Input: part model. Units: mm. Frame: model coordinates. A direction names the side the tool comes from. Coordinates: 2 decimals unless noted, no trailing zeros. Loops run counter-clockwise (first coordinate to the right, second up) from the corner with the lowest first, then second, coordinate; pieces in that order, holes last.
(1) Contact query for flat-ended pins moving along their axis: P1, Ø1.8, axis at x = -153, y = 100, coming from the +Z side; P2, Ø3, axis at x = -121, z = 4, coming from the -Y side; P3, Ø1.8, axis at x = -77.5, z = 4, coming from the +Y side. Output: stop coordinate, or through.
(2) Set-up query: faces 5 (the face through (-67, 273, 3)), 6 (the face through (-162, 136, 3)), 7 (the face through (-120, 6, 3)), 8 (the face through (-135, 96, 3)), 9 (the face through (-110.7, 271.7, 3)). Return all of +Z, -Z, +X, -X, +Y, -Y with unobstructed straight access to the full face (end or side cutting, diameter ignored); none if empty.
(3) Mould query, pull axis X, two halves, no side actions, for faces 1 (the face through (-58.7, 271.7, 3)), 2 (the face through (0, 136, 3)), 3 (the face through (-34, 276, 3)), 4 (the face through (-12.21, 5.02, 4.52)). Classes: released by +X, released by -X, zero draft, split by the parting line, or undercut.
(4) Line query: L1, parallel to Y at x = -131.5, z = 4.3; L2, parallel to Y at x = -143, z = 5.65; L3, parallel to X at y = 143, z = 1.6. Output: solid intervals per line, ascending.
(5) Section B-B, the plane y = 89. Return loops of the section in (x, z), then the cut area to 3 significant figures.
(6) Section A-A, the plane y = 178.92. Return loops of the section in (x, z).
```python
from build123d import *

# Parameters (mm, degrees)
ESQUISSE1_W             = 165
ESQUISSE1_H             = 276
BOSS_EXTRU_1_DEPTH      = 6
ESQUISSE2_W             = 38
ESQUISSE2_H             = 6
ESQUISSE2_W_2           = 6
ESQUISSE2_H_2           = 68
ESQUISSE2_W_3           = 40
EXTERIEUR_DEPTH         = 10
ESQUISSE3_R             = 11
ESQUISSE3_W             = 20
ESQUISSE3_H             = 6
ENL_V_MAT_EXTRU_2_DEPTH = 322.616230934
ESQUISSE4_R             = 1.5
ENL_V_MAT_EXTRU_3_DEPTH = 322.616230934
ESQUISSE5_R             = 2.995
ESQUISSE5_R_2           = 3
ENL_V_MAT_EXTRU_4_DEPTH = 3


with BuildPart() as part:
    # Esquisse1 → Boss.-Extru.1 (new body)
    with BuildSketch(Plane.XY):
        with Locations((-82.5, 138)):
            Rectangle(ESQUISSE1_W, ESQUISSE1_H)
    extrude(amount=BOSS_EXTRU_1_DEPTH)

    # Esquisse2 → exterieur (cut)
    with BuildSketch(Plane.XY.offset(6)):
        with Locations((-86, 273)):
            Rectangle(ESQUISSE2_W, ESQUISSE2_H)
        with Locations((-162, 238)):
            Rectangle(ESQUISSE2_W_2, ESQUISSE2_H_2)
        with Locations((-162, 102)):
            Rectangle(ESQUISSE2_W_2, ESQUISSE2_H_2)
        Polygon((-140, 36), (-140, 6), (-100, 6), (-100, 0), (-165, 0), (-165, 36), align=None)
        with Locations((-40, 3)):
            Rectangle(ESQUISSE2_W_3, ESQUISSE2_H)
    extrude(amount=-EXTERIEUR_DEPTH, mode=Mode.SUBTRACT)

    # Esquisse3 → Enlèv. mat.-Extru.2 (cut, through all)
    with BuildSketch(Plane.XY.offset(6)):
        with Locations((-144, 178.92)):
            Circle(ESQUISSE3_R)
        with Locations((-135, 99)):
            Rectangle(ESQUISSE3_W, ESQUISSE3_H)
    extrude(amount=-ENL_V_MAT_EXTRU_2_DEPTH, mode=Mode.SUBTRACT)

    # Esquisse4 → Enlèv. mat.-Extru.3 (cut, through all)
    with BuildSketch(Plane.XY.offset(6)):
        with Locations((-60, 273)):
            Circle(ESQUISSE4_R)
        with Locations((-112, 273)):
            Circle(ESQUISSE4_R)
        with Locations((-162, 197)):
            Circle(ESQUISSE4_R)
        with Locations((-162, 170)):
            Circle(ESQUISSE4_R)
        with Locations((-162, 143)):
            Circle(ESQUISSE4_R)
        with Locations((-162, 61)):
            Circle(ESQUISSE4_R)
        with Locations((-162, 43)):
            Circle(ESQUISSE4_R)
        with Locations((-93, 3)):
            Circle(ESQUISSE4_R)
        with Locations((-67, 3)):
            Circle(ESQUISSE4_R)
        with Locations((-10, 3)):
            Circle(ESQUISSE4_R)
        with Locations((-152, 99)):
            Circle(ESQUISSE4_R)
        with Locations((-118, 99)):
            Circle(ESQUISSE4_R)
    extrude(amount=-ENL_V_MAT_EXTRU_3_DEPTH, mode=Mode.SUBTRACT)

    # Esquisse5 → Enlèv. mat.-Extru.4 (cut)
    with BuildSketch(Plane.XY.offset(6)):
        with Locations((-112, 273)):
            Circle(ESQUISSE5_R)
        with Locations((-60, 273)):
            Circle(ESQUISSE5_R)
        with Locations((-162, 197)):
            Circle(ESQUISSE5_R)
        with Locations((-162, 170)):
            Circle(ESQUISSE5_R)
        with Locations((-162, 143)):
            Circle(ESQUISSE5_R)
        with Locations((-162, 61)):
            Circle(ESQUISSE5_R)
        with Locations((-162, 43)):
            Circle(ESQUISSE5_R)
        with Locations((-93, 3)):
            Circle(ESQUISSE5_R)
        with Locations((-67, 3)):
            Circle(ESQUISSE5_R)
        with Locations((-10, 3)):
            Circle(ESQUISSE5_R)
        with Locations((-152, 99)):
            Circle(ESQUISSE5_R_2)
        with Locations((-118, 99)):
            Circle(ESQUISSE5_R_2)
    extrude(amount=-ENL_V_MAT_EXTRU_4_DEPTH, mode=Mode.SUBTRACT)


solid = part.part
```
Report:
1. P1: stops at z = 3
1. P2: stops at y = 6
1. P3: stops at y = 270
2. face 5: +Z, -Z, +Y
2. face 6: +Z, -Z, -X
2. face 7: +Z, -Z, -X, -Y
2. face 8: +Z, -Z
2. face 9: +Z
3. face 1: undercut
3. face 2: released by +X
3. face 3: zero draft
3. face 4: undercut
4. L1: y = 6 to 96, 102 to 276
4. L2: y = 36 to 96, 102 to 167.97, 189.87 to 276
4. L3: x = -165 to -163.5, -160.5 to 0
5. outline: (-159, 0) - (0, 0) - (0, 6) - (-159, 6) - close
5. area: 954 mm2
6. outline: (-165, 0) - (-155, 0) - (-155, 6) - (-165, 6) - close; (-133, 0) - (0, 0) - (0, 6) - (-133, 6) - close
